from build123d import *

# Parameters (mm, degrees)
SKETCH2_R           = 15
BOSS_EXTRUDE1_DEPTH = 50
SKETCH3_W           = 10
SKETCH3_H           = 8
CUT_EXTRUDE1_DEPTH  = 60
FILLET1_R           = 5


with BuildPart() as part:
    # Sketch2 → Boss-Extrude1 (new, symmetric)
    with BuildSketch(Plane(origin=(0, 0, 0), x_dir=(-1, 0, 0), z_dir=(0, 1, 0))):
        with Locations(Location((0, 0, 0), (0, 0, 90))):
            Circle(SKETCH2_R)
    extrude(amount=BOSS_EXTRUDE1_DEPTH, both=True)

    # Sketch3 → Cut-Extrude1 (cut)
    with BuildSketch(Plane(origin=(0, 50, 0), x_dir=(-1, 0, 0), z_dir=(0, 1, 0))):
        with Locations((0, 15)):
            Rectangle(SKETCH3_W, SKETCH3_H)
    extrude(amount=-CUT_EXTRUDE1_DEPTH, mode=Mode.SUBTRACT)

    # Fillet1
    fillet1_edges = [part.edges().sort_by_distance(p)[0] for p in [
        (5, -10, 12.571067812),
        (-5, -10, 12.571067812),
    ]]
    fillet(fillet1_edges, radius=FILLET1_R - 0.0001)  # a hair under: the kernel refuses the full size


solid = part.part
Can you work these out from the model? Positions are in its coordinate system, mm. A direction names the side the tool comes from. Give positions to 0.01 mm unless a question says otherwise; leave off trailing zeros. Loops run counter-clockwise (first coordinate to the right, second up) from the corner with the lowest first, then second, coordinate; pieces in that order, holes last. Notation, with made-up numbers: M -16,7 L 26,7 A6 ccw 26,12 Z; hole C 27.5,65.5 d5. An arc over 180 degrees is marked long. One line per item, written item: value.
1) Imagine slicing it at D-D on x = 1. Write out the boundary of the cut face in (y, z).
Geometry check:
outline: M -50,-14.97 L 50,-14.97 L 50,11 L -9.9,11 L -9.9,14.97 L -50,14.97 Z
2) Imagine slicing it at B-B on x = -4. Write out the boundary of the cut face in (y, z), and give its area (3 significant figures).
Geometry check:
outline: M -50,-14.46 L 50,-14.46 L 50,11 L -8,11 L -8,14.46 L -50,14.46 Z
area: 2,690 mm²
3) I'm going to push flat-ended pins straight in: pin 1 (10 mm diameter, centred on x = 6, y = 28.5, fed in from +Z); pin 2 (0.9 mm diameter, centred on y = 33, z = 13, fed in from +X); pin 3 (12 mm diameter, centred on x = 11, y = 6.5, fed in from -Z). Where does each tip first touch, or does it pass through?
Geometry check:
pin 1: stops at z = 14.14
pin 2: stops at x = 8.22
pin 3: stops at z = -14.14
4) Imagine slicing it at C-C on z = -5.5. Write out the boundary of the cut face in (x, y), and give its area (3 significant figures).
Geometry check:
outline: M -13.96,-50 L 13.96,-50 L 13.96,50 L -13.96,50 Z
area: 2,790 mm²
5) Thinking about a two-plate mould opening in X: for faces 1 (the face through (0, 50, -1)), 2 (the face through (5, 23, 13)), 3 (the face through (0.66, 0.7, -14.985)), which applies, +X half, -X half, draft (parallel to the pull), parting line (faces both ways), or undercut?
Geometry check:
face 1: draft
face 2: undercut
face 3: parting line
6) Please list where these lines run through material, in increasing order: line 1 (X direction, y = -30.5, z = 0); line 2 (Z direction, x = -0.5, y = -32.5); line 3 (Z direction, x = 3, y = -2).
Geometry check:
line 1: x = -15 to 15
line 2: z = -14.99 to 14.99
line 3: z = -14.7 to 11
7) On a 3-axis mill with a long thin cutter (end or side, diameter ignored), from which of +Z, -Z, +X, -X, +Y, -Y can I reach the whole of each face in a straight line? I mean faces 4 (the face through (0, -50, 0)), 5 (the face through (0, 20, 11)). Say none if no direction works.
Geometry check:
face 4: +Z, -Z, +X, -X, -Y
face 5: +Z, +Y
8) Imagine slicing it at A-A on y = -19.5. Write out the boundary of the cut face in (x, z).
Geometry check:
outline: C 0,0 d30
